Answer from the drawing. Dimensions are ordinates in mm from the lowest x, y and z of the part. Give positions to 0.01 mm unless a question says otherwise; leave off trailing zeros. Loops run counter-clockwise (first coordinate to the right, second up) from the corner with the lowest first, then second, coordinate; pieces in that order, holes last.
Item 1: Section D-D, the plane z = 68.5 is taken. Give the vertices of the cut face in (x, y), and give its area (3 significant figures).
Item 2: The mould has two halves that part along Z. Classify the marked faces 1, 2 and 3: pulls with the +Z half, pulls with the -Z half, needs draft (parallel to the pull), parting line crosses it, or undercut.
Item 3: Section B-B, the plane z = 39.22 is taken. Give the vertices of the cut face in (x, y), and give its area (3 significant figures).
Item 4: Section A-A, the plane x = 39.22 is taken. Give the vertices of the cut face in (y, z), and give its area (3 significant figures).
Item 5: Consider line 1 along Z through (x, y) = (39.22, 4.75); line 2 along Z through (x, y) = (75.22, 8.5) (1 decimal); line 3 along X through (y, z) = (3.25, 24.5). Determine where each line is inside the solid, lowest interval first.
Item 6: Section C-C, the plane y = 2.5 is taken. Give the vertices of the cut face in (x, z) (1 decimal), and give its area (3 significant figures).
Item 7: Each of these flat-tipped pins is pushed along its axis until it touches: pin 1 Ø10 at (x, z) = (54.5, 50.5) entering from +Y; pin 2 Ø2 at (y, z) = (7.5, 34) entering from +X; pin 3 Ø5 at (y, z) = (6, 42.5) entering from -X. Where does it stop, or does it pass through?
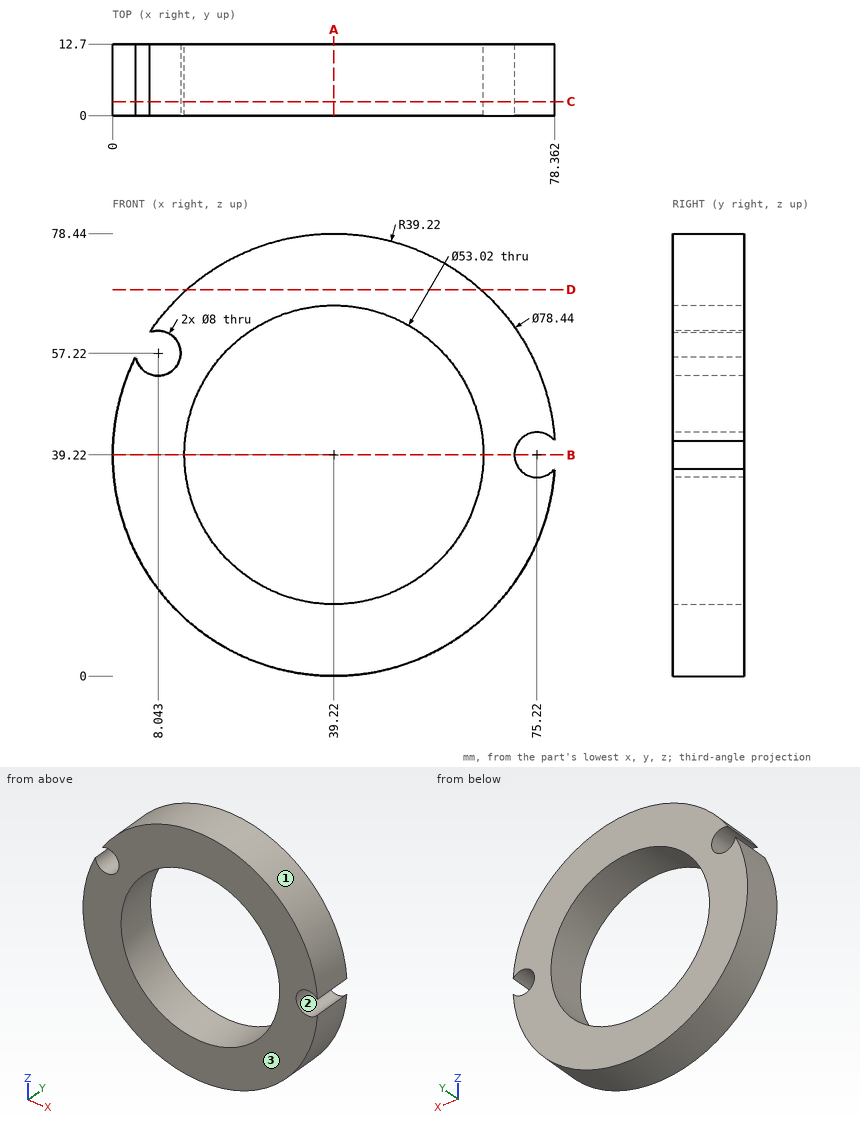
Worked answers:
1. outline: (13.13, 0) - (65.31, 0) - (65.31, 12.7) - (13.13, 12.7) - close
1. area: 663 mm2
2. face 1: pulls with the +Z half
2. face 2: undercut
2. face 3: needs draft
3. outline: (0, 0) - (12.71, 0) - (12.71, 12.7) - (0, 12.7) - close; (65.73, 0) - (71.22, 0) - (71.22, 12.7) - (65.73, 12.7) - close
3. area: 231 mm2
4. outline: (0, 0) - (12.7, 0) - (12.7, 12.71) - (0, 12.71) - close; (0, 65.73) - (12.7, 65.73) - (12.7, 78.44) - (0, 78.44) - close
4. area: 323 mm2
5. line 1: z = 0 to 12.71, 65.73 to 78.44
5. line 2: z = 23.7 to 35.2, 43.2 to 54.8
5. line 3: x = 2.87 to 17.17, 61.27 to 75.57
6. outline: (4.1, 56.6) arc R39.2 ccw (long way) to (78.4, 36.7) arc R4 cw (long way) to (78.4, 41.7) arc R39.2 ccw to (6.6, 60.9) arc R4 cw (long way) to start; hole circle Ø53 at (39.2, 39.2)
6. area: 2,530 mm2
7. pin 1: passes through
7. pin 2: stops at x = 78.21
7. pin 3: stops at x = 0.01
